Autodesk Inventor part; units mm, degrees
ref_plane "YZ Plane" through (0, 0, 0) normal (1, 0, 0) x (0, 1, 0)
ref_plane "XZ Plane" through (0, 0, 0) normal (0, 1, 0) x (-1, 0, 0)
ref_plane "XY Plane" through (0, 0, 0) normal (0, 0, 1) x (1, 0, 0)
sketch "Эскиз1" plane through (0, 0, 0) normal (0, 1, 0) x (-1, 0, 0)
  circle A0 centre (0, 0) radius 68
  dimension "d0" = 136
extrude "Выдавливание1" add sketch "Эскиз1" along normal blind 3
sketch "Эскиз2" plane through (0, 3, 0) normal (0, 1, 0) x (1, 0, 0)
  line L0 (15, -62) -> (-15, -62)
  line L1 (-15, -62) -> (-15, 62)
  line L2 (-15, 62) -> (15, 62)
  line L3 (15, 62) -> (15, -62)
  line L4 (15, -62) -> (-15, 62) construction
  line L5 (-15, -62) -> (15, 62) construction
  point P0 (0, 0)
  dimension "d3" = 30
  dimension "d4" = 124
extrude "Выдавливание2" cut sketch "Эскиз2" against normal blind 3
sketch "Эскиз3" plane through (0, 3, 0) normal (0, 1, 0) x (1, 0, 0)
  point P0 (0, 0)
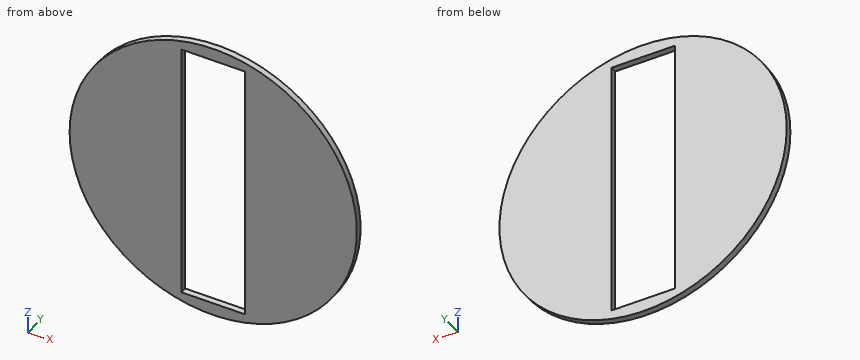
The model under review builds one solid part; all positions refer to its coordinate system, in mm. Round coordinates to 2 decimals unless told otherwise and drop trailing zeros. Loops run counter-clockwise (first coordinate to the right, second up) from the corner with the lowest first, then second, coordinate; pieces in that order, holes last. Notation, with made-up numbers: M 75.25,56 L 131.25,56 A26 cw 131.25,72 Z; hole C 80,-26 d11. An arc over 180 degrees is marked long. Answer as a JSON object with one key per item and string values.
Item 1: We need section D-D, the plane x = -39.5. State the section outline as (y, z) points, and give its area (3 significant figures).
Check sheet entries:
{"outline": "M 0,-55.35 L 3,-55.35 L 3,55.35 L 0,55.35 Z", "area": "332 mm2"}
Item 2: We need section A-A, the plane x = 0. State the section outline as (y, z) points.
Check sheet entries:
{"outline": "M 0,-68 L 3,-68 L 3,-62 L 0,-62 Z; M 0,62 L 3,62 L 3,68 L 0,68 Z"}
Item 3: We need section C-C, the plane y = 1.6. State the section outline as (x, z) points.
Check sheet entries:
{"outline": "C 0,0 d136; hole M -15,-62 L 15,-62 L 15,62 L -15,62 Z"}
Item 4: We need section B-B, the plane z = -17.5. State the section outline as (x, y) points.
Check sheet entries:
{"outline": "M -65.71,0 L -15,0 L -15,3 L -65.71,3 Z; M 15,0 L 65.71,0 L 65.71,3 L 15,3 Z"}
Item 5: For line 1 along X through (y, z) = (2.55, -22); line 2 along X through (y, z) = (2, 15); line 3 along Z through (x, y) = (-12.5, 2.2), list the stretches that pass through material, from the lowest coordinate up.
Check sheet entries:
{"line 1": "-64.34 to -15, 15 to 64.34", "line 2": "-66.32 to -15, 15 to 66.32", "line 3": "-66.84 to -62, 62 to 66.84"}
Item 6: Clearance check with flat-ended pins moving along their axes: P1, Ø0.9, axis at y = 2, z = 17, coming from the +X side; P2, Ø1, axis at x = -38.5, y = 2, coming from the +Z side; P3, Ø1.5, axis at x = -1, y = 1, coming from the -Z side. State where each tip first meets the part, or that it passes through.
Check sheet entries:
{"P1": "x = 65.96", "P2": "z = 56.39", "P3": "z = -68"}
